Geometry check sheet. Reference: the model listing, model coordinates, mm. A direction names the side the tool comes from. Round coordinates to 2 decimals unless told otherwise and drop trailing zeros. Loops run counter-clockwise (first coordinate to the right, second up) from the corner with the lowest first, then second, coordinate; pieces in that order, holes last. Notation, with made-up numbers: (40.25, 72.5) -> (91.25, 72.5) arc R18 cw to (91.25, 101.5) -> close; hole circle Ø3 at (28, -20). An arc over 180 degrees is marked (long way). Use a Markdown table: item, result. Add a question column.
Q1. Material ranges on L1, parallel to Y at x = 0, z = 1.65; L2, parallel to Z at x = -7.3, y = -17.5; L3, parallel to Z at x = -3.75, y = -17, recorded low to high.
Q2. Release check for a two-part mould opening along Y. For faces 3 (the face through (-7.48, -15.29, 21.93)), 4 (the face through (-7.479, -31.211, 13.414)), 5 (the face through (-9, -17, 10)) record: released by +Y, released by -Y, zero draft, split by the parting line, or undercut.
Q3. Sectioned sample at C-C, the plane x = -6.75. Enter the section's corners in (y, z), then the cut area to 3 significant figures.
Q4. Sectioned sample at B-B, the plane x = -4. Enter the section's corners in (y, z).
Q5. Sectioned sample at D-D, the plane z = 18.5. Enter the section's corners in (x, y), then the cut area to 3 significant figures.
Q6. Set-up check for faces 1 (the face through (-6, -17, 12)), 2 (the face through (-1.08, -4.88, 1.48)): record each of +Z, -Z, +X, -X, +Y, -Y from which the full face is reachable in a straight line by a thin tool's end or side.
Q7. Sectioned sample at A-A, the plane y = -17.5. Enter the section's corners in (x, z).
Q8. Gauge pin test, flat end, axial feed: P1, Ø2, axis at y = -31.5, z = 9.5, coming from the +X side. Record the tip position at first contact, or that the pin passes through.
```python
from build123d import *

# Parameters (mm, degrees)
F0_R     = 3
F0_R_2   = 5
F1_DEPTH = 3
F2_R     = 3
F3_DEPTH = 3
F4_R     = 5
F5_R     = 3


with BuildPart() as f1:
    # F0 (on Top) → F1 (new body)
    with BuildSketch(Plane.XY):
        Polygon((6, 6), (0, 6), (-6, 6), (-6, -41), (0, -41), (6, -41), align=None)
        with Locations((0, -35)):
            Circle(F0_R, mode=Mode.SUBTRACT)
        Circle(F0_R_2, mode=Mode.SUBTRACT)
    extrude(amount=F1_DEPTH)

    # F2 (on face) → F3 (join)
    with BuildSketch(Plane(origin=(-6, 0, 0), x_dir=(0, -1, 0), z_dir=(-1, 0, 0))):
        Polygon((17.5, 28), (-6, 3), (-6, 0), (41, 0), (41, 3), align=None)
        with Locations((17.5, 19.903563)):
            Circle(F2_R, mode=Mode.SUBTRACT)
    extrude(amount=F3_DEPTH)

    # F4
    f4_edges = [f1.edges().sort_by_distance(p)[0] for p in [
        (-7.5, -17.5, 28),
    ]]
    fillet(f4_edges, radius=F4_R)

    # F5
    f5_edges = [f1.edges().sort_by_distance(p)[0] for p in [
        (6, -41, 1.5),
        (-9, -41, 1.5),
        (6, 6, 1.5),
        (-9, 6, 1.5),
    ]]
    fillet(f5_edges, radius=F5_R)


solid = f1.part
```
Values:
| question | item | result |
|---|---|---|
| 1 | L1 | -41 to -38, -32 to -5, 5 to 6 |
| 1 | L2 | 0 to 16.9, 22.9 to 25.7 |
| 1 | L3 | 0 to 3 |
| 2 | face 3 | undercut |
| 2 | face 4 | released by -Y |
| 2 | face 5 | zero draft |
| 3 | outline | (-40.9, 0) -> (5.9, 0) -> (5.9, 3.1) -> (-13.86, 24.12) arc R5 ccw to (-21.14, 24.12) -> (-40.9, 3.1) -> close; hole circle Ø6 at (-17.5, 19.9) |
| 3 | area | 693 mm^2 |
| 4 | outline | (-41, 0) -> (-3, 0) -> (-3, 3) -> (-41, 3) -> close; (3, 0) -> (6, 0) -> (6, 3) -> (3, 3) -> close |
| 5 | outline | (-9, -26.43) -> (-6, -26.43) -> (-6, -20.15) -> (-9, -20.15) -> close; (-9, -14.85) -> (-6, -14.85) -> (-6, -8.57) -> (-9, -8.57) -> close |
| 5 | area | 37.7 mm^2 |
| 6 | face 1 | +Z, +X, +Y, -Y |
| 6 | face 2 | +Z, -Z |
| 7 | outline | (-9, 0) -> (6, 0) -> (6, 3) -> (-6, 3) -> (-6, 16.9) -> (-9, 16.9) -> close; (-9, 22.9) -> (-6, 22.9) -> (-6, 25.7) -> (-9, 25.7) -> close |
| 8 | P1 | x = -6 |
